```python
from build123d import *

# Parameters (mm, degrees)
ESQUISSE1_W             = 50
ESQUISSE1_H             = 70
ESQUISSE1_R             = 5
ESQUISSE1_R_2           = 7
ESQUISSE1_R_3           = 2.065
BASE_EXTRUSION_DEPTH    = 15
CHANFREIN3_SIZE         = 5
ENL_V_MAT_EXTRU_1_REACH = 89.321
ESQUISSE10_R            = 1.62


with BuildPart() as part:
    # Esquisse1 → Base-Extrusion (new body)
    with BuildSketch(Plane.XY):
        with Locations((0, 35)):
            Rectangle(ESQUISSE1_W, ESQUISSE1_H)
        with Locations((15, 13)):
            Circle(ESQUISSE1_R, mode=Mode.SUBTRACT)
        with Locations(Location((-15, 13, 0), (0, 0, 180))):
            Circle(ESQUISSE1_R, mode=Mode.SUBTRACT)
        with Locations((0, 35)):
            Circle(ESQUISSE1_R_2, mode=Mode.SUBTRACT)
        with Locations((-15, 60)):
            Circle(ESQUISSE1_R_3, mode=Mode.SUBTRACT)
        with Locations(Location((15, 60, 0), (0, 0, 180))):
            Circle(ESQUISSE1_R_3, mode=Mode.SUBTRACT)
    extrude(amount=BASE_EXTRUSION_DEPTH)

    # Chanfrein3
    chanfrein3_edges = [part.edges().sort_by_distance(p)[0] for p in [
        (0, 70, 0),
    ]]
    chamfer(chanfrein3_edges, length=CHANFREIN3_SIZE)

    # Esquisse10 → Enlèv. mat.-Extru.1 (cut, up to next)
    with BuildSketch(Plane(origin=(25, 0, 0), x_dir=(0, 0, -1), z_dir=(1, 0, 0)), mode=Mode.PRIVATE) as enl_v_mat_extru_1_sk1:
        with Locations((-7.5, 13)):
            Circle(ESQUISSE10_R)
    enl_v_mat_extru_1_tool1 = extrude(enl_v_mat_extru_1_sk1.sketch, amount=-ENL_V_MAT_EXTRU_1_REACH, mode=Mode.PRIVATE) & part.part
    enl_v_mat_extru_1 = enl_v_mat_extru_1_tool1.solids().sort_by_distance((25, 13, 7.5))[0]
    add(enl_v_mat_extru_1, mode=Mode.SUBTRACT)

    # Symétrie1: Enlèv. mat.-Extru.1 across plane
    add(enl_v_mat_extru_1.mirror(Plane(origin=(0, 0, 0), x_dir=(0, 0, 1), z_dir=(1, 0, 0))), mode=Mode.SUBTRACT)


solid = part.part
```
Verification items for the finished model (mm, model axes). A direction names the side the tool comes from. Give positions to 0.01 mm unless a question says otherwise; leave off trailing zeros. Write each loop counter-clockwise with the first axis right and the second up, starting at its lowest first coordinate (ties: lowest second). Pieces come first, ordered by that corner, then holes. Notation, with made-up numbers: (-35, 44) - (-17, 44) arc R23 cw to (-17, 71) - close; hole circle Ø3 at (-31.75, -11). An arc over 180 degrees is marked (long way). Put each result on its own line as item: value.
Q1. Set-up check for faces 4 (the face through (22.4, 11.42, 7.85)), 5 (the face through (14.047, 61.832, 7.395)): record each of +Z, -Z, +X, -X, +Y, -Y from which the full face is reachable in a straight line by a thin tool's end or side.
Result:
face 4: +X
face 5: +Z, -Z
Q2. Section check C-C on y = 13. Record the cut outline in (x, z), and give its area (3 significant figures).
Result:
outline: (-25, 0) - (-20, 0) - (-20, 5.88) - (-25, 5.88) - close; (-25, 9.12) - (-20, 9.12) - (-20, 15) - (-25, 15) - close; (-10, 0) - (10, 0) - (10, 15) - (-10, 15) - close; (20, 0) - (25, 0) - (25, 5.88) - (20, 5.88) - close; (20, 9.12) - (25, 9.12) - (25, 15) - (20, 15) - close
area: 418 mm2
Q3. Section check A-A on z = 12.75. Record the cut outline in (x, y) (3 decimals).
Result:
outline: (-25, 0) - (25, 0) - (25, 70) - (-25, 70) - close; hole circle Ø10 at (-15, 13); hole circle Ø4.13 at (-15, 60); hole circle Ø14 at (0, 35); hole circle Ø10 at (15, 13); hole circle Ø4.13 at (15, 60)
Q4. Section check B-B on x = 12. Record the cut outline in (y, z).
Result:
outline: (0, 0) - (9, 0) - (9, 15) - (0, 15) - close; (17, 0) - (65, 0) - (70, 5) - (70, 15) - (17, 15) - close
Q5. Mould release check, pull along Y, two halves, no side actions. Record for faces 1 (the face through (0, 0, 7)), 2 (the face through (0, 70, 10)), 3 (the face through (-22.4, 11.42, 7.85)): released by +Y, released by -Y, zero draft, split by the parting line, or undercut.
Result:
face 1: released by -Y
face 2: released by +Y
face 3: undercut
Q6. Section check D-D on z = 7.5. Record the cut outline in (x, y) (3 decimals).
Result:
outline: (-25, 0) - (25, 0) - (25, 11.38) - (19.73, 11.38) arc R5 cw (long way) to (19.73, 14.62) - (25, 14.62) - (25, 70) - (-25, 70) - (-25, 14.62) - (-19.73, 14.62) arc R5 cw (long way) to (-19.73, 11.38) - (-25, 11.38) - close; hole circle Ø4.13 at (-15, 60); hole circle Ø14 at (0, 35); hole circle Ø4.13 at (15, 60)
Q7. Scan lines: probe 1 along Y at (x, z) = (15, 9.75) (3 decimals); probe 2 along Y at (x, z) = (-22.8, 7.5); probe 3 along Y at (x, z) = (0, 5). Record each from-to range of solid material in increasing order. Write a range as from..to.
Result:
probe 1: 0..8, 18..57.935, 62.065..70
probe 2: 0..11.38, 14.62..70
probe 3: 0..28, 42..70
Q8. Depth check by flat-ended pin: P1, Ø8, axis at x = -15, y = 13, coming from the +Z side; P2, Ø3.5, axis at y = 13, z = 7.5, coming from the +X side; P3, Ø1.9, axis at y = 13, z = 7.5, coming from the -X side. Enter the tip coordinate at first touch or a pass-through.
Result:
P1: through
P2: x = 25
P3: x = -10.09
